```python
from build123d import *

# Parameters (mm, degrees)
SKETCH_1_R           = 0.75
EXTRUDE_1_DEPTH      = 0.5
EXTRUDE_1_DEPTH_BACK = 0.5


with BuildPart() as part:
    # Sketch 1 → Extrude 1 (new body, two sides)
    with BuildSketch(Plane(origin=(0, 0, 0), x_dir=(0, 0, -1), z_dir=(1, 0, 0))) as extrude_1_sk:
        with BuildLine():
            Line((-3.95, -6.512622113), (-3.95, -7.25))
            ThreePointArc((-3.95, -7.25), (-3.452081528, -8.452081528), (-2.25, -8.95))
            Line((-2.25, -8.95), (-0.45, -8.95))
            Line((-0.45, -8.95), (-0.45, -5.732364259))
            ThreePointArc((-0.45, -5.732364259), (0, 5.75), (0.45, -5.732364259))
            Line((0.45, -5.732364259), (0.45, -8.95))
            Line((0.45, -8.95), (2.25, -8.95))
            ThreePointArc((2.25, -8.95), (3.452081528, -8.452081528), (3.95, -7.25))
            Line((3.95, -7.25), (3.95, -6.512622113))
            ThreePointArc((3.95, -6.512622113), (4.117151006, -5.777520785), (4.585734072, -5.186975842))
            ThreePointArc((4.585734072, -5.186975842), (0, 7.85), (-4.585734072, -5.186975842))
            ThreePointArc((-4.585734072, -5.186975842), (-4.117151006, -5.777520785), (-3.95, -6.512622113))
        make_face()
        with Locations((2.2, -7.25)):
            Circle(SKETCH_1_R, mode=Mode.SUBTRACT)
        with Locations((-2.2, -7.25)):
            Circle(SKETCH_1_R, mode=Mode.SUBTRACT)
    extrude(amount=EXTRUDE_1_DEPTH)
    extrude(extrude_1_sk.sketch, amount=-EXTRUDE_1_DEPTH_BACK)


solid = part.part
```
Part model, mm, in its own coordinate system. A direction names the side the tool comes from. Round coordinates to 2 decimals unless told otherwise and drop trailing zeros. Write each loop counter-clockwise with the first axis right and the second up, starting at its lowest first coordinate (ties: lowest second). Pieces come first, ordered by that corner, then holes.
Item 1: Cut at C-C, the plane y = 0.25. Give the cut face in (x, z), plus the area to 3 significant figures.
Results:
outline: (-0.5, -7.32) - (0.5, -7.32) - (0.5, -5.74) - (-0.5, -5.74) - close; (-0.5, 5.74) - (0.5, 5.74) - (0.5, 7.32) - (-0.5, 7.32) - close
area: 3.15 mm2
Item 2: Drop flat-ended pins along their axis: pin 1 Ø1.5 at (y, z) = (4.5, 2) entering from +X; pin 2 Ø0.5 at (x, y) = (0, -7) entering from -Z; pin 3 Ø0.5 at (x, y) = (0, -7) entering from +Z. Give the stop position or say it passes through.
Results:
pin 1: passes through
pin 2: stops at z = -3.95
pin 3: stops at z = 3.95
Item 3: Two-plate mould, pull along Y, no slides. Class faces 3 (the cylindrical face through (-0.01, -7.22, -1.45)), 4 (the flat face through (0, -8.95, -1)), 5 (the cylindrical face through (0.007, 5.745, 0.247)), 6 (the flat face through (0, -7, 0.45)): +Y half, -Y half, draft (parallel to the pull), parting line (faces both ways), or undercut.
Results:
face 3: undercut
face 4: -Y half
face 5: undercut
face 6: draft
Item 4: Cut at A-A, the plane y = -7. Give the cut face in (x, z).
Results:
outline: (-0.5, -3.95) - (0.5, -3.95) - (0.5, -2.91) - (-0.5, -2.91) - close; (-0.5, -1.49) - (0.5, -1.49) - (0.5, -0.45) - (-0.5, -0.45) - close; (-0.5, 0.45) - (0.5, 0.45) - (0.5, 1.49) - (-0.5, 1.49) - close; (-0.5, 2.91) - (0.5, 2.91) - (0.5, 3.95) - (-0.5, 3.95) - close
Item 5: Cut at B-B, the plane z = 3.25. Give the cut face in (x, y), plus the area to 3 significant figures.
Results:
outline: (-0.5, -8.62) - (0.5, -8.62) - (0.5, -4.74) - (-0.5, -4.74) - close; (-0.5, 4.74) - (0.5, 4.74) - (0.5, 7.09) - (-0.5, 7.09) - close
area: 6.23 mm2
Item 6: Which spindle directions (+Z, -Z, +X, -X, +Y, -Y) get a long thin tool onto all of the face, cutting with end or side? Do faces 1 (the cylindrical face through (0, -8.4, 3.5)), 2 (the flat face through (0, -7, -0.45)). Say none if no direction does.
Results:
face 1: +Z, +X, -X, -Y
face 2: +X, -X, -Y
Item 7: Probe L1, parallel to Y at x = 0.2, z = 1.75; L2, parallel to Y at x = -0.15, z = 0; L3, parallel to Z at x = -0.35, y = -4.25. List the from-to ranges inside material, lowest first.
Results:
L1: y = -8.95 to -7.85, -6.65 to -5.48, 5.48 to 7.64
L2: y = 5.75 to 7.85
L3: z = -5.55 to -3.87, 3.87 to 5.55
Item 8: Cut at D-D, the plane z = -6.5. Give the cut face in (x, y).
Results:
outline: (-0.5, -2.85) - (0.5, -2.85) - (0.5, 3.9) - (-0.5, 3.9) - close
